The model under review builds one solid part; all positions refer to its coordinate system, in mm. A direction names the side the tool comes from. Coordinates: 2 decimals unless noted, no trailing zeros. Order: outer loops, then holes, each group sorted by start corner. A loop starts at its lowest first (then second) coordinate and runs counter-clockwise, first axis right, second up.
```python
from build123d import *

# Parameters (mm, degrees)
BOSS_EXTRUDE2_DEPTH = 3.5
CUT_EXTRUDE1_DEPTH  = 6


with BuildPart() as part:
    # Sketch4 → Boss-Extrude2 (new body)
    with BuildSketch(Plane.XY):
        Polygon((30.881516436, 14.964687786), (16.881516436, 14.964687786), (16.881516436, 16.964687786), (14.381516436, 16.964687786), (14.381516436, 19.884687786), (20.702643433, 19.884687786), (30.881516436, 19.884687786), (30.881516436, 16.964687786), align=None)
    extrude(amount=BOSS_EXTRUDE2_DEPTH)

    # Sketch5 → Cut-Extrude1 (cut)
    with BuildSketch(Plane(origin=(0, 19.884687786, 0), x_dir=(1, 0, 0), z_dir=(0, 1, 0))):
        with BuildLine():
            Line((27.881516436, -3.5), (29.881516436, -3.5))
            ThreePointArc((29.881516436, -3.5), (27.881516436, -1.5), (25.881516436, -3.5))
            Line((25.881516436, -3.5), (27.881516436, -3.5))
        make_face()
    extrude(amount=-CUT_EXTRUDE1_DEPTH, mode=Mode.SUBTRACT)


solid = part.part
```
(1) We need section A-A, the plane z = 3.25. Write out the cut boundary in (x, y), and give its area (3 significant figures).
A:
outline: (14.38, 16.96) - (16.88, 16.96) - (16.88, 14.96) - (25.9, 14.96) - (25.9, 19.88) - (14.38, 19.88) - close; (29.87, 14.96) - (30.88, 14.96) - (30.88, 19.88) - (29.87, 19.88) - close
area: 56.7 mm2
(2) Machinability: for faces 1 (the face through (16.882, 16, 2)), 2 (the face through (30.882, 17, 2)), which of the approach directions +Z, -Z, +X, -X, +Y, -Y give a long, thin tool a straight path to every point of the face, cutting with its end or side? Answer none if there is none.
A:
face 1: +Z, -Z, -X, -Y
face 2: +Z, -Z, +X, +Y, -Y
(3) For pin 1 Ø0.6 at (y, z) = (16.5, 1.5) entering from -X, flat-tipped, find the tip position at first contact; note if it passes through.
A:
pin 1: stops at x = 16.88
(4) Draft analysis for pull direction Z (two halves, no side actions). For faces 3 (the face through (14.382, 18, 2)), 4 (the face through (20, 17, 3.5)), 5 (the face through (23, 17, 0)), state which applies: released by +Z, released by -Z, zero draft, split by the parting line, or undercut.
A:
face 3: zero draft
face 4: released by +Z
face 5: released by -Z
(5) We need section D-D, the plane x = 15.5. Write out the cut boundary in (y, z), and give its area (3 significant figures).
A:
outline: (16.96, 0) - (19.88, 0) - (19.88, 3.5) - (16.96, 3.5) - close
area: 10.2 mm2
(6) We need section C-C, the plane z = 1.1. Write out the cut boundary in (x, y).
A:
outline: (14.38, 16.96) - (16.88, 16.96) - (16.88, 14.96) - (30.88, 14.96) - (30.88, 19.88) - (14.38, 19.88) - close
(7) Wall thickness on probe 1 along X at (y, z) = (16.7, 0.85); probe 2 along X at (y, z) = (17.1, 3.25); probe 3 along Y at (x, z) = (15.75, 2.8): over which ranges is each line inside the solid? List them lowest first.
A:
probe 1: x = 16.88 to 30.88
probe 2: x = 14.38 to 25.9, 29.87 to 30.88
probe 3: y = 16.96 to 19.88
(8) We need section B-B, the plane y = 15.9. Write out the cut boundary in (x, z), and give its area (3 significant figures).
A:
outline: (16.88, 0) - (30.88, 0) - (30.88, 3.5) - (29.88, 3.5) arc R2 cw to (25.88, 3.5) - (16.88, 3.5) - close
area: 42.7 mm2
